Part model, mm, in its own coordinate system. Give positions to 0.01 mm unless a question says otherwise; leave off trailing zeros. Order: outer loops, then holes, each group sorted by start corner. A loop starts at its lowest first (then second) coordinate and runs counter-clockwise, first axis right, second up. Notation, with made-up numbers: M 44,49.25 L 53,49.25 A18 ccw 53,55.25 Z; hole C -10,19.25 d3. An arc over 180 degrees is marked long. Answer as a JSON object with one key per item and string values.
from build123d import *

# Parameters (mm, degrees)
F0_W      = 40
F0_H      = 40
F1_DEPTH  = 600
F2_R      = 3
F3_DEPTH  = 12
F4_R      = 3
F5_DEPTH  = 12
F6_R      = 3
F7_DEPTH  = 22
F8_W      = 15
F8_H      = 440
F9_DEPTH  = 10
F10_W     = 15
F10_H     = 440
F11_DEPTH = 10


with BuildPart() as f1:
    # F0 (on Top) → F1 (new body)
    with BuildSketch(Plane.XY):
        with Locations((20, -20)):
            Rectangle(F0_W, F0_H)
    extrude(amount=F1_DEPTH)

    # F2 (on face) → F3 (cut)
    with BuildSketch(Plane.YZ.offset(40)):
        with Locations((-20, 570)):
            Circle(F2_R)
    extrude(amount=-F3_DEPTH, mode=Mode.SUBTRACT)

    # F4 (on face) → F5 (cut)
    with BuildSketch(Plane(origin=(0, 0, 0), x_dir=(-1, 0, 0), z_dir=(0, 1, 0))):
        with Locations((-20, 570)):
            Circle(F4_R)
    extrude(amount=-F5_DEPTH, mode=Mode.SUBTRACT)

    # F6 (on face) → F7 (cut)
    with BuildSketch(Plane.XY.offset(600)):
        with Locations((20, -20)):
            Circle(F6_R)
    extrude(amount=-F7_DEPTH, mode=Mode.SUBTRACT)

    # F8 (on face) → F9 (cut)
    with BuildSketch(Plane.XZ.offset(40)):
        with Locations((20, 300)):
            Rectangle(F8_W, F8_H)
    extrude(amount=-F9_DEPTH, mode=Mode.SUBTRACT)

    # F10 (on face) → F11 (cut)
    with BuildSketch(Plane(origin=(0, 0, 0), x_dir=(0, -1, 0), z_dir=(-1, 0, 0))):
        with Locations((20, 300)):
            Rectangle(F10_W, F10_H)
    extrude(amount=-F11_DEPTH, mode=Mode.SUBTRACT)


solid = f1.part
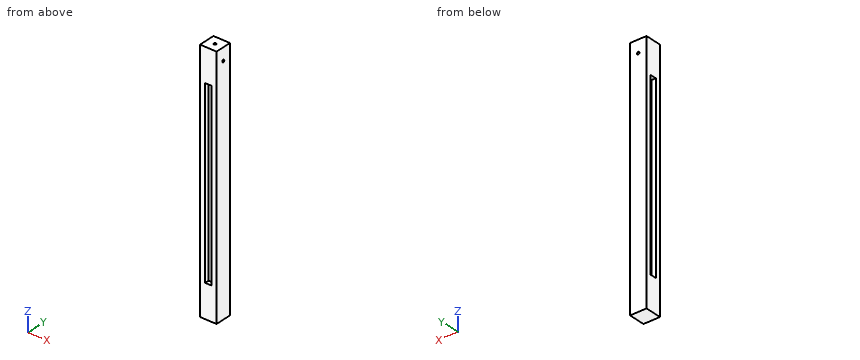
1. Probe line 1 along Y through (x, z) = (35, 570); line 2 along Z through (x, y) = (8, -24); line 3 along X through (y, z) = (-38, 508.5). List the from-to ranges inside material, lowest first.
Worked answers:
{"line 1": "y = -40 to -23, -17 to 0", "line 2": "z = 0 to 80, 520 to 600", "line 3": "x = 0 to 12.5, 27.5 to 40"}
2. Pin check, flat tips, straight feed: P1, Ø7.5, axis at x = 21.5, z = 224.5, coming from the -Y side; P2, Ø5, axis at y = -24, z = 184, coming from the -X side. Stop position of each tip, or through.
Worked answers:
{"P1": "stops at y = -30", "P2": "stops at x = 10"}
3. Cut at A-A on z = 446.5. Give the cut face in (x, y), plus the area to 3 significant figures.
Worked answers:
{"outline": "M 0,-40 L 12.5,-40 L 12.5,-30 L 27.5,-30 L 27.5,-40 L 40,-40 L 40,0 L 0,0 L 0,-12.5 L 10,-12.5 L 10,-27.5 L 0,-27.5 Z", "area": "1,300 mm^2"}
